Geometry check sheet. Reference: drawing and pictorial views, mm from the part's lowest x, y, z. A direction names the side the tool comes from. Coordinates: 2 decimals unless noted, no trailing zeros. Loops run counter-clockwise (first coordinate to the right, second up) from the corner with the lowest first, then second, coordinate; pieces in that order, holes last. Notation, with made-up numbers: (-37, 64.25) -> (11, 64.25) arc R12 ccw to (11, 81.25) -> close; hole circle Ø4 at (-13, 86.25). An arc over 180 degrees is marked (long way). Answer as a JSON object with one key per item and string values.
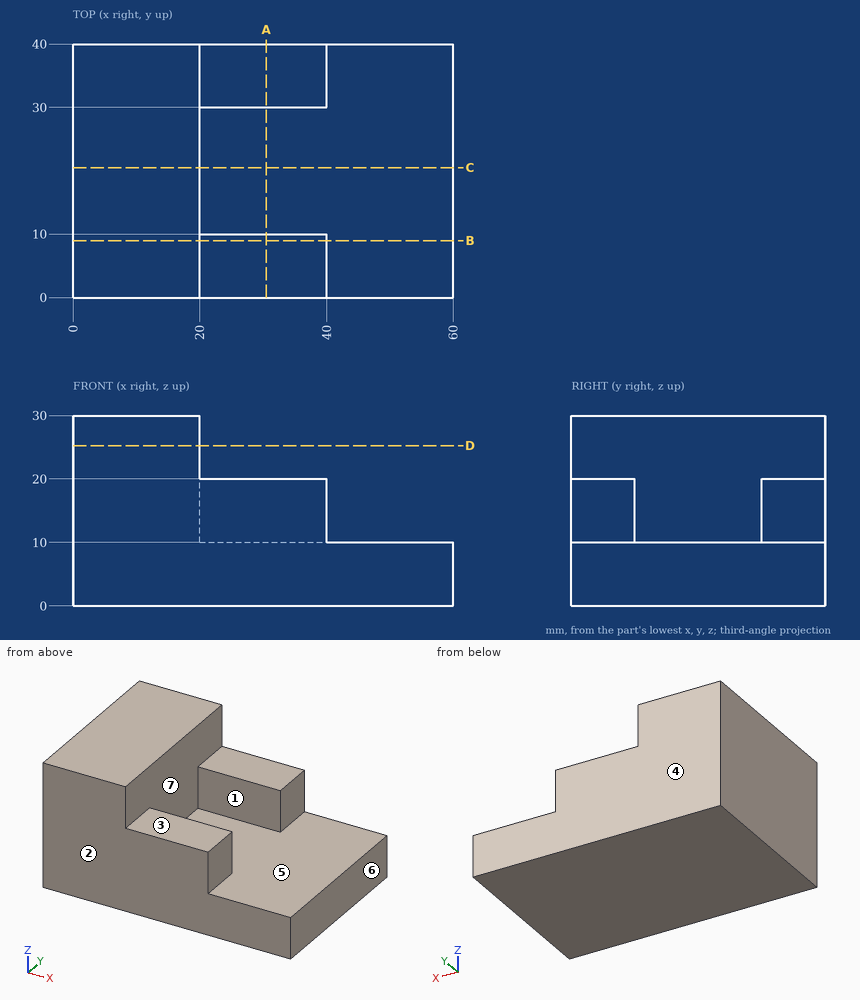
1. Thickness scan on probe 1 along Y at (x, z) = (28, 13.5); probe 2 along X at (y, z) = (25, 17.25); probe 3 along Z at (x, y) = (30, 18.5). Record the ranges inside material, lowest first. Write a range as from..to.
Evaluation:
{"probe 1": "y = 0..10, 30..40", "probe 2": "x = 0..20", "probe 3": "z = 0..10"}
2. Tool access check on the marked faces 1, 2 and 3. Record the directions out of +Z, -Z, +X, -X, +Y, -Y that give a thin tool (end or side, any length) a straight path to the whole face; none if there is none.
Evaluation:
{"face 1": "+Z, +X", "face 2": "+Z, -Z, +X, -X, -Y", "face 3": "+Z, +X, +Y, -Y"}
3. Depth check by flat-ended pin: P1, Ø3, axis at y = 6.5, z = 16.5, coming from the +X side; P2, Ø5, axis at x = 34.5, y = 3, coming from the +Z side; P3, Ø6, axis at y = 15, z = 16.5, coming from the +X side; P4, Ø2, axis at x = 47.5, y = 27, coming from the -Z side. Enter the tip coordinate at first touch or a pass-through.
Evaluation:
{"P1": "stops at x = 40", "P2": "stops at z = 20", "P3": "stops at x = 20", "P4": "stops at z = 0"}
4. Mould release check, pull along Y, two halves, no side actions. Record for the marked faces 4, 5, 6 and 7: released by +Y, released by -Y, zero draft, split by the parting line, or undercut.
Evaluation:
{"face 4": "released by +Y", "face 5": "undercut", "face 6": "zero draft", "face 7": "undercut"}
5. Section check C-C, the plane y = 20.5. Record the boundary of the cut face in (x, z), then the cut area to 3 significant figures.
Evaluation:
{"outline": "(0, 0) -> (60, 0) -> (60, 10) -> (20, 10) -> (20, 30) -> (0, 30) -> close", "area": "1,000 mm^2"}
6. Section check D-D, the plane z = 25.25. Record the boundary of the cut face in (x, y), then the cut area to 3 significant figures.
Evaluation:
{"outline": "(0, 0) -> (20, 0) -> (20, 40) -> (0, 40) -> close", "area": "800 mm^2"}
7. Section check A-A, the plane x = 30.5. Record the boundary of the cut face in (y, z).
Evaluation:
{"outline": "(0, 0) -> (40, 0) -> (40, 20) -> (30, 20) -> (30, 10) -> (10, 10) -> (10, 20) -> (0, 20) -> close"}
8. Section check B-B, the plane y = 9. Record the boundary of the cut face in (x, z).
Evaluation:
{"outline": "(0, 0) -> (60, 0) -> (60, 10) -> (40, 10) -> (40, 20) -> (20, 20) -> (20, 30) -> (0, 30) -> close"}
